from build123d import *

# Parameters (mm, degrees)
CROQUIS1_W              = 240
CROQUIS1_H              = 260
SALIENTE_EXTRUIR1_DEPTH = 15
CROQUIS6_R              = 2.55
CORTAR_EXTRUIR3_DEPTH   = 178.552809046
CROQUIS7_R              = 5.5
CORTAR_EXTRUIR4_DEPTH   = 5
CROQUIS8_R              = 3.5
CORTAR_EXTRUIR5_DEPTH   = 178.552809046


with BuildPart() as part:
    # Croquis1 → Saliente-Extruir1 (new body)
    with BuildSketch(Plane(origin=(0, 0, 0), x_dir=(1, 0, 0), z_dir=(0, 1, 0))):
        Rectangle(CROQUIS1_W, CROQUIS1_H)
    extrude(amount=SALIENTE_EXTRUIR1_DEPTH)

    # Croquis6 → Cortar-Extruir3 (cut, through all)
    with BuildSketch(Plane.XZ):
        with Locations(Location((-45.5, -47.5, 0), (0, 0, 270))):
            Circle(CROQUIS6_R)
        with Locations(Location((-97.5, -47.5, 0), (0, 0, 270))):
            Circle(CROQUIS6_R)
        with Locations(Location((-97.5, 47.5, 0), (0, 0, 270))):
            Circle(CROQUIS6_R)
        with Locations(Location((-45.5, 47.5, 0), (0, 0, 270))):
            Circle(CROQUIS6_R)
        with Locations(Location((45.5, 47.5, 0), (0, 0, 270))):
            Circle(CROQUIS6_R)
        with Locations(Location((97.5, 47.5, 0), (0, 0, 270))):
            Circle(CROQUIS6_R)
        with Locations(Location((45.5, -47.5, 0), (0, 0, 270))):
            Circle(CROQUIS6_R)
        with Locations(Location((97.5, -47.5, 0), (0, 0, 270))):
            Circle(CROQUIS6_R)
    extrude(amount=-CORTAR_EXTRUIR3_DEPTH, mode=Mode.SUBTRACT)

    # Croquis7 → Cortar-Extruir4 (cut)
    with BuildSketch(Plane(origin=(0, 15, 0), x_dir=(1, 0, 0), z_dir=(0, 1, 0))):
        with Locations(Location((-97.5, 47.5, 0), (0, 0, 270))):
            Circle(CROQUIS7_R)
        with Locations(Location((-45.5, 47.5, 0), (0, 0, 270))):
            Circle(CROQUIS7_R)
        with Locations(Location((-97.5, -47.5, 0), (0, 0, 270))):
            Circle(CROQUIS7_R)
        with Locations(Location((-45.5, -47.5, 0), (0, 0, 270))):
            Circle(CROQUIS7_R)
        with Locations(Location((45.5, -47.5, 0), (0, 0, 270))):
            Circle(CROQUIS7_R)
        with Locations(Location((97.5, -47.5, 0), (0, 0, 270))):
            Circle(CROQUIS7_R)
        with Locations(Location((97.5, 47.5, 0), (0, 0, 270))):
            Circle(CROQUIS7_R)
        with Locations(Location((45.5, 47.5, 0), (0, 0, 270))):
            Circle(CROQUIS7_R)
    extrude(amount=-CORTAR_EXTRUIR4_DEPTH, mode=Mode.SUBTRACT)

    # Croquis8 → Cortar-Extruir5 (cut, through all)
    with BuildSketch(Plane(origin=(0, 15, 0), x_dir=(1, 0, 0), z_dir=(0, 1, 0))):
        with Locations(Location((-100, 100, 0), (0, 0, 270))):
            Circle(CROQUIS8_R)
        with Locations(Location((-50, 100, 0), (0, 0, 270))):
            Circle(CROQUIS8_R)
        with Locations(Location((0, 100, 0), (0, 0, 270))):
            Circle(CROQUIS8_R)
        with Locations(Location((50, 100, 0), (0, 0, 270))):
            Circle(CROQUIS8_R)
        with Locations(Location((100, 100, 0), (0, 0, 270))):
            Circle(CROQUIS8_R)
        with Locations(Location((0, 50, 0), (0, 0, 270))):
            Circle(CROQUIS8_R)
        with Locations(Location((-50, 0, 0), (0, 0, 270))):
            Circle(CROQUIS8_R)
        with Locations(Location((0, 0, 0), (0, 0, 270))):
            Circle(CROQUIS8_R)
        with Locations(Location((50, 0, 0), (0, 0, 270))):
            Circle(CROQUIS8_R)
        with Locations(Location((100, 0, 0), (0, 0, 270))):
            Circle(CROQUIS8_R)
        with Locations(Location((0, -50, 0), (0, 0, 270))):
            Circle(CROQUIS8_R)
        with Locations(Location((-50, -100, 0), (0, 0, 270))):
            Circle(CROQUIS8_R)
        with Locations(Location((0, -100, 0), (0, 0, 270))):
            Circle(CROQUIS8_R)
        with Locations(Location((50, -100, 0), (0, 0, 270))):
            Circle(CROQUIS8_R)
        with Locations(Location((100, -100, 0), (0, 0, 270))):
            Circle(CROQUIS8_R)
        with Locations(Location((-100, 0, 0), (0, 0, 270))):
            Circle(CROQUIS8_R)
        with Locations(Location((-100, -100, 0), (0, 0, 270))):
            Circle(CROQUIS8_R)
    extrude(amount=-CORTAR_EXTRUIR5_DEPTH, mode=Mode.SUBTRACT)


solid = part.part
Can you work these out from the model? Positions are in its coordinate system, mm. A direction names the side the tool comes from. Coordinates: 2 decimals unless noted, no trailing zeros. Write each loop counter-clockwise with the first axis right and the second up, starting at its lowest first coordinate (ties: lowest second). Pieces come first, ordered by that corner, then holes. Notation, with made-up numbers: (84.25, -15) -> (99.25, -15) arc R19 cw to (99.25, 22) -> close; hole circle Ø1 at (14.25, 30). An arc over 180 degrees is marked (long way). Answer as CSV lines item,"result".
1) If we section it at C-C on x = 0: Please give me the cut outline in (y, z), then the cut area to 4 significant figures.
Check result:
outline,"(0, -130) -> (15, -130) -> (15, -103.5) -> (0, -103.5) -> close; (0, -96.5) -> (15, -96.5) -> (15, -53.5) -> (0, -53.5) -> close; (0, -46.5) -> (15, -46.5) -> (15, -3.5) -> (0, -3.5) -> close; (0, 3.5) -> (15, 3.5) -> (15, 46.5) -> (0, 46.5) -> close; (0, 53.5) -> (15, 53.5) -> (15, 96.5) -> (0, 96.5) -> close; (0, 103.5) -> (15, 103.5) -> (15, 130) -> (0, 130) -> close"
area,"3,375 mm²"
2) If we mould it in two halves opening along X, with no side actions, what happens to faces 1 (the flat face through (-120, 7, 2)), 2 (the cylindrical face through (-101.341, 7.605, -96.767)), 3 (the flat face through (-48, 10, 49)), 4 (the flat face through (-28, 15, -2))? For each: +X half, -X half, draft (parallel to the pull), parting line (faces both ways), or undercut.
Check result:
face 1,"-X half"
face 2,"undercut"
face 3,"undercut"
face 4,"draft"
3) If we section it at B-B on y = 12.5: Count the separate pieces of the cut face and the enclosed holes in it, then the cut area to 3 significant figures.
Check result:
separate pieces,"1"
enclosed holes,"25"
area,"61,000 mm²"
4) If I drill on line 1 (Z direction, x = 52.5, y = 5.75); line 2 (X direction, y = 7.5, z = 0); line 3 (X direction, y = 12.1, z = 47.5), over which ranges is the centre line in solid material (lowest first)? Write a range as from..to.
Check result:
line 1,"-130..-102.45, -97.55..-2.45, 2.45..97.55, 102.45..130"
line 2,"-120..-103.5, -96.5..-53.5, -46.5..-3.5, 3.5..46.5, 53.5..96.5, 103.5..120"
line 3,"-120..-103, -92..-51, -40..-2.45, 2.45..40, 51..92, 103..120"
5) Will this pin go through, and if not, where does the flat tip stop? P1, Ø6, axis at x = 97.5, z = 47.5, coming from the +Y side.
Check result:
P1,"y = 10"
6) On a 3-axis mill with a long thin cutter (end or side, diameter ignored), from which of +Z, -Z, +X, -X, +Y, -Y can I reach the whole of each face in a straight line? I mean faces 5 (the flat face through (95, 10, 49)), 6 (the cylindrical face through (53.47, 7.6, -0.46)). Say none if no direction works.
Check result:
face 5,"+Y"
face 6,"+Y, -Y"
7) If we section it at A-A on z = 100: Please give me the cut outline in (x, y).
Check result:
outline,"(-120, 0) -> (-103.5, 0) -> (-103.5, 15) -> (-120, 15) -> close; (-96.5, 0) -> (-53.5, 0) -> (-53.5, 15) -> (-96.5, 15) -> close; (-46.5, 0) -> (-3.5, 0) -> (-3.5, 15) -> (-46.5, 15) -> close; (3.5, 0) -> (46.5, 0) -> (46.5, 15) -> (3.5, 15) -> close; (53.5, 0) -> (96.5, 0) -> (96.5, 15) -> (53.5, 15) -> close; (103.5, 0) -> (120, 0) -> (120, 15) -> (103.5, 15) -> close"
